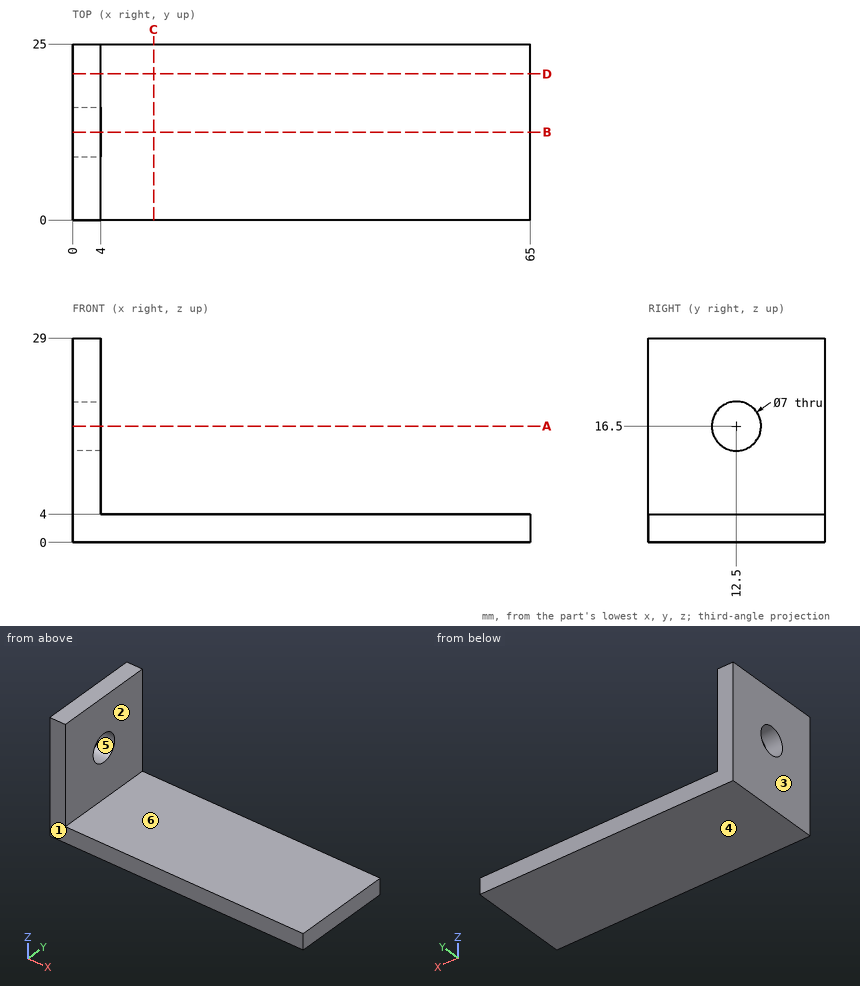
Check sheet for the drawn part. Datum: minimum x, y, z corner. Units: mm. A direction names the side the tool comes from. Round coordinates to 2 decimals unless told otherwise and drop trailing zeros. Order: outer loops, then holes, each group sorted by start corner. A loop starts at its lowest first (then second) coordinate and runs counter-clockwise, first axis right, second up. Notation, with made-up numbers: M 81.5,-36.75 L 96.5,-36.75 A28 cw 96.5,-15.75 Z; hole C -14,-13 d11. An arc over 180 degrees is marked long. Answer in a Markdown table with one row per item.
(1) Draft check along Z on the marked faces 3, 4, 5 and 6. Enter one of: +Z half, -Z half, draft (parallel to the pull), parting line (faces both ways), or undercut.
Findings:
| item | result |
|---|---|
| face 3 | draft |
| face 4 | -Z half |
| face 5 | undercut |
| face 6 | +Z half |
(2) Section check B-B on y = 12.5. Record the boundary of the cut face in (x, z), plus the area to 3 significant figures.
Findings:
| item | result |
|---|---|
| outline | M 0,0 L 65,0 L 65,4 L 4,4 L 4,13 L 0,13 Z; M 0,20 L 4,20 L 4,29 L 0,29 Z |
| area | 332 mm^2 |
(3) Gauge pin test, flat ends, axial feed: pin 1 (4 mm diameter, centred on y = 12.5, z = 16.5, fed in from -X); pin 2 (7.5 mm diameter, centred on y = 9.5, z = 16.5, fed in from +X); pin 3 (1.5 mm diameter, centred on x = 22, y = 15.5, fed in from +Z). Record the tip position at first contact, or that the pin passes through.
Findings:
| item | result |
|---|---|
| pin 1 | passes through |
| pin 2 | stops at x = 4 |
| pin 3 | stops at z = 4 |
(4) Set-up check for the marked faces 1 and 2: record each of +Z, -Z, +X, -X, +Y, -Y from which the full face is reachable in a straight line by a thin tool's end or side.
Findings:
| item | result |
|---|---|
| face 1 | +Z, -Z, +X, -X, -Y |
| face 2 | +Z, +X, +Y, -Y |
(5) Section check D-D on y = 20.75. Record the boundary of the cut face in (x, z), plus the area to 3 significant figures.
Findings:
| item | result |
|---|---|
| outline | M 0,0 L 65,0 L 65,4 L 4,4 L 4,29 L 0,29 Z |
| area | 360 mm^2 |
(6) Section check A-A on z = 16.5. Record the boundary of the cut face in (x, y).
Findings:
| item | result |
|---|---|
| outline | M 0,0 L 4,0 L 4,9 L 0,9 Z; M 0,16 L 4,16 L 4,25 L 0,25 Z |
(7) Material ranges on line 1 along Y through (x, z) = (2.2, 16.5); line 2 along X through (y, z) = (22, 22.5), recorded low to high. Write a range as from..to.
Findings:
| item | result |
|---|---|
| line 1 | y = 0..9, 16..25 |
| line 2 | x = 0..4 |
(8) Section check C-C on x = 11.5. Record the boundary of the cut face in (y, z), plus the area to 3 significant figures.
Findings:
| item | result |
|---|---|
| outline | M 0,0 L 25,0 L 25,4 L 0,4 Z |
| area | 100 mm^2 |
